Read the model definition and answer for the solid it produces. Units are mm, in the model's axes. A direction names the side the tool comes from. Coordinates: 2 decimals unless noted, no trailing zeros. Loops run counter-clockwise (first coordinate to the right, second up) from the corner with the lowest first, then second, coordinate; pieces in that order, holes last.
from build123d import *

# Parameters (mm, degrees)
F1_DEPTH = 9
F4_DEPTH = 21


with BuildPart() as f1:
    # F0 (on Top) → F1 (new body)
    with BuildSketch(Plane.XY):
        with BuildLine():
            Line((51, 30), (0, 30))
            ThreePointArc((0, 30), (-15, 15), (0, 0))
            Line((0, 0), (51, 0))
            Line((51, 0), (60, 9))
            Line((60, 9), (60, 21))
            Line((60, 21), (51, 30))
        make_face()
    extrude(amount=F1_DEPTH)

    # F2 (on face) → F4 (join)
    with BuildSketch(Plane.XY.offset(9)):
        with BuildLine():
            Line((18, 30), (0, 30))
            ThreePointArc((0, 30), (-15, 15), (0, 0))
            Line((0, 0), (18, 0))
            Line((18, 0), (18, 30))
        make_face()
    extrude(amount=F4_DEPTH)


solid = f1.part
Item 1: Given pin 1 (5 mm diameter, centred on y = 24.5, z = 18.5, fed in from +X); pin 2 (8 mm diameter, centred on y = 25.5, z = 7, fed in from -X); pin 3 (10 mm diameter, centred on y = 25, z = 11.5, fed in from -X), each flat-ended and moving along its own axis, determine where each tip first touches the part or whether it passes through.
Numbers:
pin 1: stops at x = 18
pin 2: stops at x = -13.52
pin 3: stops at x = -14.14
Item 2: Which of the six approach directions +Z, -Z, +X, -X, +Y, -Y give full straight-line access (tool end or side, diameter ignored) to faces 1 (the face through (-15, 15, 15)), 2 (the face through (18, 15, 19))?
Numbers:
face 1: +Z, -Z, -X
face 2: +Z, +X, +Y, -Y
Item 3: Find the intervals of material crossed by line 1 along Z through (x, y) = (55.5, 15); line 2 along X through (y, z) = (14.5, 24.5); line 3 along X through (y, z) = (22.25, 13), in increasing order.
Numbers:
line 1: z = 0 to 9
line 2: x = -14.99 to 18
line 3: x = -13.13 to 18
Item 4: A cutting plane is placed at D-D on z = 14. Determine the outline of the cut face in (x, y), then the cut area to 3 significant figures.
Numbers:
outline: (0, 0) - (18, 0) - (18, 30) - (0, 30) arc R15 ccw to start
area: 893 mm2
Item 5: A cutting plane is placed at C-C on x = 23. Determine the outline of the cut face in (y, z).
Numbers:
outline: (0, 0) - (30, 0) - (30, 9) - (0, 9) - close
Item 6: A cutting plane is placed at A-A on z = 7.75. Determine the outline of the cut face in (x, y), then the cut area to 3 significant figures.
Numbers:
outline: (0, 0) - (51, 0) - (60, 9) - (60, 21) - (51, 30) - (0, 30) arc R15 ccw to start
area: 2,070 mm2
Item 7: A cutting plane is placed at B-B on y = 15. Determine the outline of the cut face in (x, z).
Numbers:
outline: (-15, 0) - (60, 0) - (60, 9) - (18, 9) - (18, 30) - (-15, 30) - close
